The listing builds one solid part. Answer for the finished solid, in the listing's coordinates (mm). Coordinates: 2 decimals unless noted, no trailing zeros. Order: outer loops, then holes, each group sorted by start corner. A loop starts at its lowest first (then second) coordinate and runs counter-clockwise, first axis right, second up.
from build123d import *

# Parameters (mm, degrees)
SKETCH_F_W                   = 449
SKETCH_F_H                   = 84
SKETCH_F_R                   = 2
SKETCH_F_W_2                 = 70
SKETCH_F_H_2                 = 35
ESTRUSIONE_ESTRUSIONE1_DEPTH = 3


with BuildPart() as part:
    # Sketch f → Estrusione-Estrusione1 (new body)
    with BuildSketch(Plane.XY):
        with Locations((224.5, 42)):
            Rectangle(SKETCH_F_W, SKETCH_F_H)
        with Locations((9, 42)):
            Circle(SKETCH_F_R, mode=Mode.SUBTRACT)
        with Locations((224.5, 75)):
            Circle(SKETCH_F_R, mode=Mode.SUBTRACT)
        with Locations((224.5, 9)):
            Circle(SKETCH_F_R, mode=Mode.SUBTRACT)
        with Locations((440, 42)):
            Circle(SKETCH_F_R, mode=Mode.SUBTRACT)
        with Locations((334, 75)):
            Circle(SKETCH_F_R, mode=Mode.SUBTRACT)
        with Locations((334, 9)):
            Circle(SKETCH_F_R, mode=Mode.SUBTRACT)
        with Locations(Location((115, 9, 0), (0, 0, 180))):
            Circle(SKETCH_F_R, mode=Mode.SUBTRACT)
        with Locations(Location((115, 75, 0), (0, 0, 180))):
            Circle(SKETCH_F_R, mode=Mode.SUBTRACT)
        with Locations((369, 42)):
            Rectangle(SKETCH_F_W_2, SKETCH_F_H_2, mode=Mode.SUBTRACT)
    extrude(amount=ESTRUSIONE_ESTRUSIONE1_DEPTH)


solid = part.part
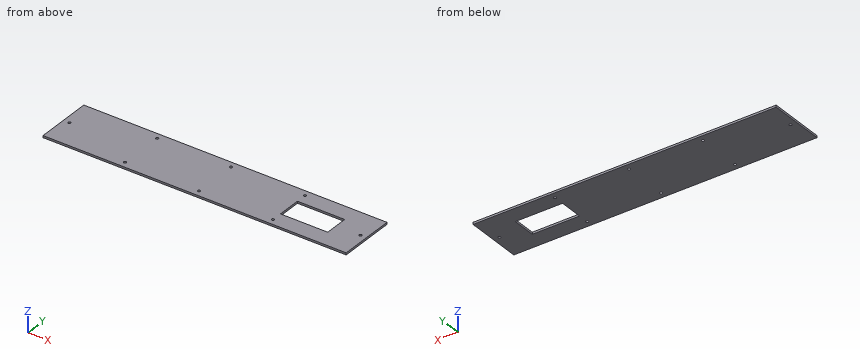
1) Section A-A (z = 2.1) is taken. Give the number of separate pieces and of enclosed holes in the cut face, then the cut area to 3 significant figures.
2) Section B-B (y = 33.5) is taken. Give the vertices of the cut face in (x, z), then the cut area to 3 significant figures.
3) Consider L1, parallel to Y at x = 115, z = 0.9; L2, parallel to X at y = 36, z = 1.05; L3, parallel to X at y = 8.5, z = 0.6. Determine where each line is inside the solid, lowest interval first.
4) This flat-tipped pin is pushed along its axis until it touches: P1, Ø3.5, axis at x = 334, y = 75, coming from the -Z side. Where does it stop, or does it pass through?
Filled sheet:
1. separate pieces: 1
1. enclosed holes: 9
1. area: 35,200 mm2
2. outline: (0, 0) - (334, 0) - (334, 3) - (0, 3) - close; (404, 0) - (449, 0) - (449, 3) - (404, 3) - close
2. area: 1,140 mm2
3. L1: y = 0 to 7, 11 to 73, 77 to 84
3. L2: x = 0 to 334, 404 to 449
3. L3: x = 0 to 113.06, 116.94 to 222.56, 226.44 to 332.06, 335.94 to 449
4. P1: passes through
